Geometry: final body of the model. Coordinates: model frame, mm. Face numbers are marked on the shaded views. A direction names the side the tool comes from. Coordinates: 2 decimals unless noted, no trailing zeros. Loops run counter-clockwise (first coordinate to the right, second up) from the corner with the lowest first, then second, coordinate; pieces in that order, holes last. Notation, with made-up numbers: (-13, 41) - (-1, 41) arc R8 cw to (-1, 56) - close; hole circle Ø2 at (-29, 21.25). An arc over 180 degrees is marked (long way). Return JSON: item names as keys, results as strings.
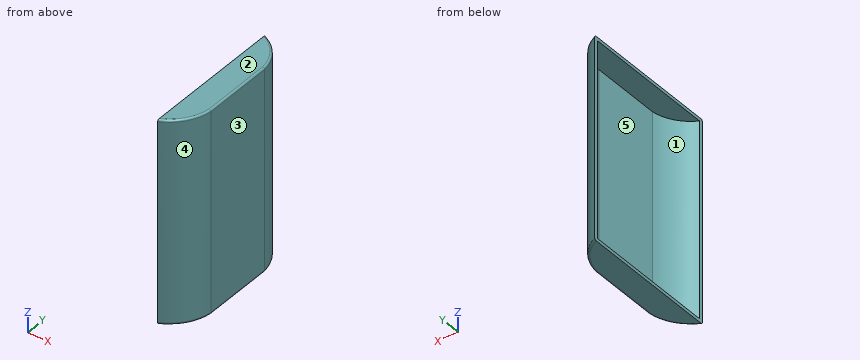
from build123d import *

# Parameters (mm, degrees)
MAIN_SHAPE_DEPTH = 110.6
HOLLOW_T         = -1.8
FILLETS_R        = 1


with BuildPart() as part:
    # Sketch for the main shape → Main shape (new body)
    with BuildSketch(Plane.XY):
        with BuildLine():
            Line((14.361069392, 19.95), (14.361069392, 59.95))
            ThreePointArc((14.361069392, 59.95), (9.818254591, 71.823770849), (0, 79.9))
            Line((0, 79.9), (0, 0))
            ThreePointArc((0, 0), (9.818254591, 8.076229151), (14.361069392, 19.95))
        make_face()
    extrude(amount=MAIN_SHAPE_DEPTH)

    # Hollow
    hollow_openings = [part.faces().sort_by_distance(p)[0] for p in [
        (0, 39.95, 55.3),
    ]]
    offset(amount=HOLLOW_T, openings=hollow_openings, kind=Kind.INTERSECTION)

    # Fillets
    # the kernel refuses this fillet: 1 mm, written as the material it takes off along each edge
    with BuildSketch(Plane(origin=(-10.361710586, 57.297160312, 110.6), x_dir=(0.9999799478441757, 0.006332764764284822, 0), z_dir=(0.006332764764284822, -0.9999799478441757, 0))) as fillets_piece_1:
        with BuildLine():
            CenterArc((24.864702054 - FILLETS_R, -FILLETS_R), FILLETS_R, 0, 90)
            Line((24.864702054 - FILLETS_R, 0), (24.864702054, 0))
            Line((24.864702054, 0), (24.864702054, -FILLETS_R))
        make_face()
    revolve(axis=Axis((-10.361710586, 57.297160312, 110.6), (0, 0, 1)), revolution_arc=70.771001335, mode=Mode.SUBTRACT)
    with BuildSketch(Plane(origin=(-10.361710586, 22.602839688, 110.6), x_dir=(0.32335851179223435, -0.9462765308573977, 0), z_dir=(-0.9462765308573977, -0.32335851179223435, 0))) as fillets_piece_2:
        with BuildLine():
            CenterArc((24.864702054 - FILLETS_R, -FILLETS_R), FILLETS_R, 0, 90)
            Line((24.864702054 - FILLETS_R, 0), (24.864702054, 0))
            Line((24.864702054, 0), (24.864702054, -FILLETS_R))
        make_face()
    revolve(axis=Axis((-10.361710586, 22.602839688, 110.6), (0, 0, 1)), revolution_arc=70.771001335, mode=Mode.SUBTRACT)
    with BuildSketch(Plane(origin=(-10.361710586, 57.297160312, 0), x_dir=(0.9999799478441757, 0.006332764764284822, 0), z_dir=(0.006332764764284822, -0.9999799478441757, 0))) as fillets_piece_3:
        with BuildLine():
            CenterArc((24.864702054 - FILLETS_R, FILLETS_R), FILLETS_R, 270, 90)
            Line((24.864702054 - FILLETS_R, 0), (24.864702054, 0))
            Line((24.864702054, 0), (24.864702054, FILLETS_R))
        make_face()
    revolve(axis=Axis((-10.361710586, 57.297160312, 0), (0, 0, 1)), revolution_arc=70.771001335, mode=Mode.SUBTRACT)
    with BuildSketch(Plane(origin=(14.361069392, 17.45, 0), x_dir=(0, 0, 1), z_dir=(0, 1, 0))) as fillets_piece_4:
        with BuildLine():
            CenterArc((FILLETS_R, -FILLETS_R), FILLETS_R, 90, 90)
            Line((0, -FILLETS_R), (0, 0))
            Line((0, 0), (FILLETS_R, 0))
        make_face()
    extrude(amount=45, mode=Mode.SUBTRACT)
    with BuildSketch(Plane(origin=(-10.361710586, 22.602839688, 0), x_dir=(0.32335851179223435, -0.9462765308573977, 0), z_dir=(-0.9462765308573977, -0.32335851179223435, 0))) as fillets_piece_5:
        with BuildLine():
            CenterArc((24.864702054 - FILLETS_R, FILLETS_R), FILLETS_R, 270, 90)
            Line((24.864702054 - FILLETS_R, 0), (24.864702054, 0))
            Line((24.864702054, 0), (24.864702054, FILLETS_R))
        make_face()
    revolve(axis=Axis((-10.361710586, 22.602839688, 0), (0, 0, 1)), revolution_arc=70.771001335, mode=Mode.SUBTRACT)
    with BuildSketch(Plane(origin=(14.361069392, 17.45, 110.6), x_dir=(0, 0, -1), z_dir=(0, 1, 0))) as fillets_piece_6:
        with BuildLine():
            CenterArc((FILLETS_R, FILLETS_R), FILLETS_R, 180, 90)
            Line((0, FILLETS_R), (0, 0))
            Line((0, 0), (FILLETS_R, 0))
        make_face()
    extrude(amount=45, mode=Mode.SUBTRACT)


solid = part.part
Item 1: Reachability of the marked faces 1 and 2 from +Z, -Z, +X, -X, +Y, -Y: full face, straight path, thin tool, end or side. Return the list, or none.
Worked out:
{"face 1": "-X", "face 2": "+Z, +X, -X, +Y, -Y"}
Item 2: Mould query, pull axis Y, two halves, no side actions, for the marked faces 3, 4 and 5. Classes: +Y half, -Y half, draft (parallel to the pull), parting line (faces both ways), or undercut.
Worked out:
{"face 3": "draft", "face 4": "-Y half", "face 5": "undercut"}
Item 3: First-contact query: pin 1 Ø1.5 at (x, z) = (11.5, 46.5) entering from +Y; pin 2 Ø10 at (y, z) = (46, 65) entering from -X. Flat tips, straight axial feed; report the tip coordinate or a pass-through.
Worked out:
{"pin 1": "y = 70.43", "pin 2": "x = 12.56"}
Item 4: Ray query, probe 1 along Z at (x, y) = (9, 65); probe 2 along Z at (x, y) = (13.5, 45.5); probe 3 along Y at (x, z) = (11, 4). Return the intervals inside material, ascending. Write a range as from..to.
Worked out:
{"probe 1": "0..1.8, 108.8..110.6", "probe 2": "0.01..110.59", "probe 3": "9.88..13.9, 66..70.02"}
Item 5: Section query A-A, the plane z = 28.5. Return loops of the section in (x, y), and give its area (3 significant figures).
Worked out:
{"outline": "(0, 0) arc R24.86 ccw to (14.36, 19.95) - (14.36, 59.95) arc R24.86 ccw to (0, 79.9) - (0, 77.9) arc R23.06 cw to (12.56, 59.85) - (12.56, 20.05) arc R23.06 cw to (0, 2) - close", "area": "159 mm^2"}
Item 6: Section query B-B, the plane y = 40. Return loops of the section in (x, z).
Worked out:
{"outline": "(0, 0) - (13.36, 0) arc R1 ccw to (14.36, 1) - (14.36, 109.6) arc R1 ccw to (13.36, 110.6) - (0, 110.6) - (0, 108.8) - (12.56, 108.8) - (12.56, 1.8) - (0, 1.8) - close"}
